from build123d import *


with BuildPart() as f1:
    # F0 (on Front) → F1 (revolve)
    with BuildSketch(Plane.XZ):
        Polygon((-97.82505, 25.938069), (-62.771387, 25.201321), (34.941703, 25.201321), (46.073571, 25.205852), (76.681621, 25.21831), (76.681621, 41.68978), (34.941703, 41.68978), (34.941703, 52.412558), (7.590632, 52.412558), (7.590632, 77.59431), (-28.9685, 77.59431), (-28.9685, 52.412558), (-62.771387, 52.412558), (-62.771387, 42.655021), (-97.82505, 42.655021), align=None)
    revolve(axis=Axis((11.750303, 0, 0), (1, 0, 0)))


solid = f1.part
The listing builds one solid part. Answer for the finished solid, in the listing's coordinates (mm). A direction names the side the tool comes from. Give positions to 0.01 mm unless a question says otherwise; leave off trailing zeros. Write each loop counter-clockwise with the first axis right and the second up, starting at its lowest first coordinate (ties: lowest second). Pieces come first, ordered by that corner, then holes.
1) For a pull along Z with two mould halves and no side action, classify faces 4 (the face through (-80.053, -7.679, 24.384)), 5 (the face through (-13.231, -17.032, -18.574)), 6 (the face through (55.519, -41.335, -5.427)), 7 (the face through (7.591, 51, -16)) as pulls with the +Z half, pulls with the -Z half, needs draft (parallel to the pull), parting line crosses it, or undercut.
2) Section A-A (x = -8) is taken. Write down the section's boundary in (y, z), and give its area (3 significant figures).
3) Section B-B (z = -39) is taken. Write down the section's boundary in (x, y).
4) A tool of negligible diameter and unlimited length cuts with its end or side. For faces 1 (the face through (-62.771, 42.5, 7.5)), 2 (the face through (-10.94, -23.31, 74.01)), 3 (the face through (21.075, 51.166, -11.362)), from which of +Z, -Z, +X, -X, +Y, -Y can it reach the whole face along a straight path? Write none if from no direction.
5) Section D-D (z = 34) is taken. Write down the section's boundary in (x, y).
6) Section C-C (x = -39) is taken. Write down the section's boundary in (y, z).
7) Given P1, Ø4, axis at y = 7, z = 52.5, coming from the +X side; P2, Ø4, axis at x = 37, y = 19, coming from the +Z side; P3, Ø6, axis at y = 53.5, z = -50, coming from the +X side, each flat-ended and moving along its own axis, determine where each tip first touches the part or whether it passes through.
8) Find the intervals of material crossed by L1, parallel to Z at x = -25, y = 0; L2, parallel to Z at x = -39, y = 0, in increasing order.
Response:
1. face 4: undercut
1. face 5: undercut
1. face 6: parting line crosses it
1. face 7: needs draft
2. outline: circle Ø155.19 at (0, 0); hole circle Ø50.4 at (0, 0)
2. area: 16,900 mm2
3. outline: (-97.83, -17.28) - (-62.77, -17.28) - (-62.77, -35.02) - (-28.97, -35.02) - (-28.97, -67.08) - (7.59, -67.08) - (7.59, -35.02) - (34.94, -35.02) - (34.94, -14.73) - (76.68, -14.73) - (76.68, 14.73) - (34.94, 14.73) - (34.94, 35.02) - (7.59, 35.02) - (7.59, 67.08) - (-28.97, 67.08) - (-28.97, 35.02) - (-62.77, 35.02) - (-62.77, 17.28) - (-97.83, 17.28) - close
4. face 1: -X
4. face 2: +X, -X
4. face 3: +X
5. outline: (-97.83, -25.76) - (-62.77, -25.76) - (-62.77, -39.89) - (-28.97, -39.89) - (-28.97, -69.75) - (7.59, -69.75) - (7.59, -39.89) - (34.94, -39.89) - (34.94, -24.13) - (76.68, -24.13) - (76.68, 24.13) - (34.94, 24.13) - (34.94, 39.89) - (7.59, 39.89) - (7.59, 69.75) - (-28.97, 69.75) - (-28.97, 39.89) - (-62.77, 39.89) - (-62.77, 25.76) - (-97.83, 25.76) - close
6. outline: circle Ø104.83 at (0, 0); hole circle Ø50.4 at (0, 0)
7. P1: stops at x = 34.94
7. P2: stops at z = 38.07
7. P3: stops at x = 7.59
8. L1: z = -77.59 to -25.2, 25.2 to 77.59
8. L2: z = -52.41 to -25.2, 25.2 to 52.41
